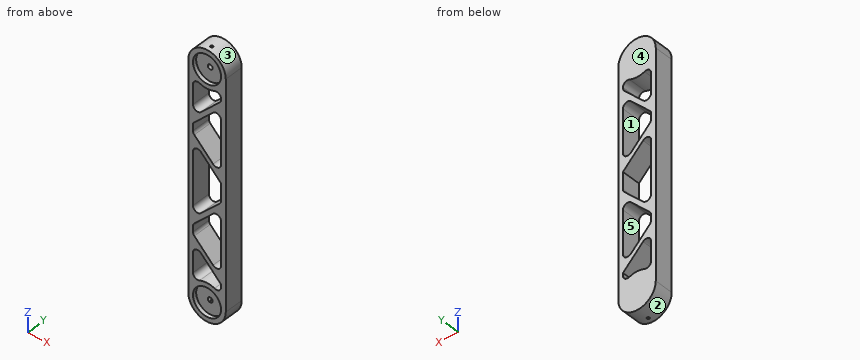
from build123d import *

# Parameters (mm, degrees)
SKETCH1_R           = 12.7
BOSS_EXTRUDE1_DEPTH = 12.7
SKETCH2_R           = 1.6256
CUT_EXTRUDE1_DEPTH  = 9.525
SKETCH3_R           = 9.525
CUT_EXTRUDE2_DEPTH  = 2.54
BOSS_EXTRUDE2_START = -12.7
BOSS_EXTRUDE2_DEPTH = 12.7
SKETCH10_R          = 1.651
CUT_EXTRUDE4_DEPTH  = 9.525
SKETCH11_R          = 9.525
CUT_EXTRUDE5_DEPTH  = 2.54
CUT_EXTRUDE6_DEPTH  = 12.7
FILLET1_R           = 3.175


with BuildPart() as part:
    # Sketch1 → Boss-Extrude1 (new body)
    with BuildSketch(Plane(origin=(0, 0, 0), x_dir=(1, 0, 0), z_dir=(0, 1, 0))):
        with Locations(Location((0, 0, 0), (0, 0, 270))):
            Circle(SKETCH1_R)
    extrude(amount=BOSS_EXTRUDE1_DEPTH)

    # Sketch2 → Cut-Extrude1 (cut)
    with BuildSketch(Plane.XZ):
        with Locations(Location((0, 0, 0), (0, 0, 270))):
            Circle(SKETCH2_R)
    extrude(amount=-CUT_EXTRUDE1_DEPTH, mode=Mode.SUBTRACT)

    # Sketch3 → Cut-Extrude2 (cut)
    with BuildSketch(Plane.XZ):
        with Locations(Location((0, 0, 0), (0, 0, 270))):
            Circle(SKETCH3_R)
    extrude(amount=-CUT_EXTRUDE2_DEPTH, mode=Mode.SUBTRACT)

    # Sketch5 → #2-56 Tapped Hole1 (revolve, cut)
    with BuildSketch(Plane(origin=(0, 3.81, 0), x_dir=(0, 1, 0), z_dir=(1, 0, 0))):
        Polygon((0, 0), (0, 13.74216509), (0.889, 13.208), (0.889, 0), align=None)
    revolve(axis=Axis((0, 3.81, -6.35), (0, 0, 1)), mode=Mode.SUBTRACT)

    # Sketch7 → Boss-Extrude2 (add)
    with BuildSketch(Plane(origin=(0, 12.7, 0), x_dir=(1, 0, 0), z_dir=(0, 1, 0)).offset(BOSS_EXTRUDE2_START)):
        with BuildLine():
            Line((-12.7, 152.4), (-12.7, 0))
            ThreePointArc((-12.7, 0), (0, 12.7), (12.7, 0))
            Line((12.7, 0), (12.7, 152.4))
            ThreePointArc((12.7, 152.4), (0, 165.1), (-12.7, 152.4))
        make_face()
    extrude(amount=BOSS_EXTRUDE2_DEPTH)

    # Sketch10 → Cut-Extrude4 (cut)
    with BuildSketch(Plane.XZ):
        with Locations(Location((0, -152.4, 0), (0, 0, 270))):
            Circle(SKETCH10_R)
    extrude(amount=-CUT_EXTRUDE4_DEPTH, mode=Mode.SUBTRACT)

    # Sketch11 → Cut-Extrude5 (cut)
    with BuildSketch(Plane.XZ):
        with Locations(Location((0, -152.4, 0), (0, 0, 270))):
            Circle(SKETCH11_R)
    extrude(amount=-CUT_EXTRUDE5_DEPTH, mode=Mode.SUBTRACT)

    # Sketch14 → #2-56 Tapped Hole2 (revolve, cut)
    with BuildSketch(Plane(origin=(0, 3.81, -152.4), x_dir=(0, -1, 0), z_dir=(1, 0, 0))):
        Polygon((0, 0), (0, 13.74216509), (0.889, 13.208), (0.889, 0), align=None)
    revolve(axis=Axis((0, 3.81, -146.05), (0, 0, -1)), mode=Mode.SUBTRACT)

    # Sketch15 → Cut-Extrude6 (cut)
    with BuildSketch(Plane.XZ):
        with BuildLine():
            Line((-9.525, -35.469743879), (9.525, -16.419743879))
            Line((9.525, -16.419743879), (9.525, -8.400260413))
            ThreePointArc((9.525, -8.400260413), (0, -12.7), (-9.525, -8.400260413))
            Line((-9.525, -8.400260413), (-9.525, -35.469743879))
        make_face()
        Polygon((-9.525, -46.309871939), (9.525, -65.359871939), (9.525, -20.909871939), (-9.525, -39.959871939), align=None)
        Polygon((-9.525, -76.2), (9.525, -76.2), (9.525, -69.85), (-9.525, -50.8), align=None)
        Polygon((9.525, -82.55), (9.525, -76.2), (-9.525, -76.2), (-9.525, -101.6), align=None)
        Polygon((9.525, -131.490128061), (9.525, -87.040128061), (-9.525, -106.090128061), (-9.525, -112.440128061), align=None)
        with BuildLine():
            Line((9.525, -143.999739587), (9.525, -135.980256121))
            Line((9.525, -135.980256121), (-9.525, -116.930256121))
            Line((-9.525, -116.930256121), (-9.525, -143.999739587))
            ThreePointArc((-9.525, -143.999739587), (0, -139.7), (9.525, -143.999739587))
        make_face()
    extrude(amount=-CUT_EXTRUDE6_DEPTH, mode=Mode.SUBTRACT)

    # Fillet1
    fillet1_edges = [part.edges().sort_by_distance(p)[0] for p in [
        (9.525, 6.35, -143.999739587),
        (-9.525, 6.35, -143.999739587),
        (-9.525, 6.35, -116.930256121),
        (-9.525, 6.35, -35.469743879),
        (9.525, 6.35, -16.419743879),
        (9.525, 6.35, -8.400260413),
        (-9.525, 6.35, -8.400260413),
        (-9.525, 6.35, -46.309871939),
        (9.525, 6.35, -65.359871939),
        (9.525, 6.35, -20.909871939),
        (-9.525, 6.35, -101.6),
        (-9.525, 6.35, -50.8),
        (9.525, 6.35, -82.55),
        (9.525, 6.35, -131.490128061),
        (9.525, 6.35, -87.040128061),
        (-9.525, 6.35, -106.090128061),
        (-9.525, 6.35, -112.440128061),
    ]]
    fillet(fillet1_edges, radius=FILLET1_R)


solid = part.part
Could you check a few things on this model? Use its own coordinates, in mm. Face numbers are marked on the shaded views. A direction names the side the tool comes from. Round coordinates to 2 decimals unless told otherwise and drop trailing zeros. Write each loop counter-clockwise with the first axis right and the second up, starting at its lowest first coordinate (ties: lowest second). Pieces come first, ordered by that corner, then holes. Notation, with made-up numbers: (30, 44.25) -> (34, 44.25) arc R27 cw to (34, 80.25) -> close; hole circle Ø1 at (15.5, -40). An arc over 180 degrees is marked (long way). Use a Markdown table: item, result.
1. If we section it at A-A (z = -79.5): List the corners of the cut face in (x, y) for me (3 decimals), then the cut area to 3 significant figures.
Answer key:
| item | result |
|---|---|
| outline | (-12.7, 0) -> (-9.525, 0) -> (-9.525, 12.7) -> (-12.7, 12.7) -> close; (9.525, 0) -> (12.7, 0) -> (12.7, 12.7) -> (9.525, 12.7) -> close |
| area | 80.6 mm^2 |
2. We'd pull the mould along Z, two halves only. Please class the marked faces 3, 4 and 5: +Z half, -Z half, draft (parallel to the pull), parting line (faces both ways), or undercut.
Answer key:
| item | result |
|---|---|
| face 3 | +Z half |
| face 4 | draft |
| face 5 | undercut |
3. Which directions (+Z, -Z, +X, -X, +Y, -Y) give clear straight access to the entire face, cutting with the end or side of a thin tool? Please do the marked faces 1 and 2.
Answer key:
| item | result |
|---|---|
| face 1 | +Y, -Y |
| face 2 | -Z, +Y, -Y |
4. Please list where these lines run through material, in increasing order: probe 1 along Z at (x, y) = (-1, 11) (3 decimals); probe 2 along X at (y, z) = (1.2, 0) (3 decimals); probe 3 along X at (y, z) = (4.25, -152.4).
Answer key:
| item | result |
|---|---|
| probe 1 | z = -165.061 to -139.739, -125.455 to -120.965, -97.565 to -93.075, -59.325 to -54.835, -31.435 to -26.945, -12.661 to 12.661 |
| probe 2 | x = -12.7 to -9.525, 9.525 to 12.7 |
| probe 3 | x = -12.7 to -1.65, 1.65 to 12.7 |
5. For pin 1 Ø3.5 at (x, z) = (0, -151.5) entering from -Y; pin 2 Ø1.1 at (x, y) = (0, 3.81) entering from -Z; pin 3 Ø3 at (x, z) = (0, 0) entering from -Y (3 decimals), each with a flat end and sliding along its axis, tell me the tip position at first contact or that it passes through.
Answer key:
| item | result |
|---|---|
| pin 1 | stops at y = 2.54 |
| pin 2 | stops at z = -150.84 |
| pin 3 | stops at y = 9.525 |
6. If we section it at B-B (x = 7): State how many separate pieces and enclosed holes the cut face has, then the cut area to 3 significant figures.
Answer key:
| item | result |
|---|---|
| separate pieces | 6 |
| enclosed holes | 0 |
| area | 825 mm^2 |
